Read the model definition and answer for the solid it produces. Units are mm, in the model's axes. Face numbers are marked on the shaded views. A direction names the side the tool comes from. Coordinates: 2 decimals unless noted, no trailing zeros. Order: outer loops, then holes, each group sorted by start corner. A loop starts at its lowest first (then second) coordinate and runs counter-clockwise, first axis right, second up. Notation, with made-up numbers: (28, -3) - (65, -3) arc R21 ccw to (65, 26) - close; hole circle Ø3 at (-29, 48). An arc over 180 degrees is marked (long way). Use one line per item in the form item = value. Start each with the question number.
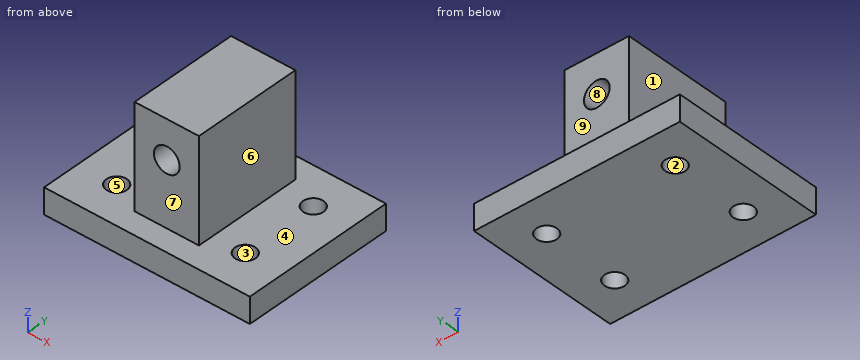
from build123d import *

# Parameters (mm, degrees)
F0_W     = 50.8
F0_H     = 38.1
F1_DEPTH = 6.35
F2_W     = 15.875
F2_H     = 27
F3_DEPTH = 25.4
F4_R     = 3.175
F5_DEPTH = 32.551
F7_D     = 5.0546


with BuildPart() as f1:
    # F0 (on Top) → F1 (new body)
    with BuildSketch(Plane.XY):
        Rectangle(F0_W, F0_H)
    extrude(amount=F1_DEPTH)

    # F2 (on face) → F3 (join)
    with BuildSketch(Plane.XY.offset(6.35)):
        Rectangle(F2_W, F2_H)
    extrude(amount=F3_DEPTH)

    # F4 (on face) → F5 (cut, through all)
    with BuildSketch(Plane.XZ.offset(13.5)):
        with Locations((0, 22.225)):
            Circle(F4_R)
    extrude(amount=-F5_DEPTH, mode=Mode.SUBTRACT)

    # F7 (through all)
    with Locations(Plane.XY.offset(6.35)):
        with Locations((-15.875, 9.525), (-15.875, -9.525), (15.875, 9.525), (15.875, -9.525)):
            Hole(F7_D / 2)


solid = f1.part
Q1. Which of the six approach directions +Z, -Z, +X, -X, +Y, -Y give full straight-line access (tool end or side, diameter ignored) to the marked faces 5, 6, 7, 8 and 9?
Q2. A cutting plane is placed at A-A (x = 0). Give the vertices of the cut face in (y, z).
Q3. A cutting plane is placed at C-C (z = 2). Give the vertices of the cut face in (x, y) (3 decimals), then the cut area to 3 significant figures.
Q4. Given P1, Ø4.5, axis at x = -15.875, y = -9.525, coming from the +Z side; P2, Ø8, axis at x = -2, z = 16, coming from the +Y side; P3, Ø8.5, axis at x = 0, z = 22.225, coming from the -Y side; P4, Ø3, axis at x = 14, y = 1.5, coming from the +Z side, each flat-ended and moving along its own axis, determine where each tip first touches the part or whether it passes through.
Q5. A cutting plane is placed at B-B (y = 8.5). Give the number of separate pieces and of enclosed holes in the cut face, then the cut area to 3 significant figures.
Q6. For a pull along X with two mould halves and no side action, classify the marked faces 1, 2, 3 and 4 as +X half, -X half, draft (parallel to the pull), parting line (faces both ways), or undercut.
Q7. Consider probe 1 along Z at (x, y) = (0, -1); probe 2 along X at (y, z) = (3.5, 12.5); probe 3 along Y at (x, z) = (-5, 8.5). Determine where each line is inside the solid, lowest interval first.
Q8. A cutting plane is placed at D-D (y = -15). Give the vertices of the cut face in (x, z), then the cut area to 3 significant figures.
Result sheet:
q1.face_5 = +Z, -Z
q1.face_6 = +Z, +X, +Y, -Y
q1.face_7 = +Z, +X, -X, -Y
q1.face_8 = +Y, -Y
q1.face_9 = +Z, +X, -X, +Y
q2.outline = (-19.05, 0) - (19.05, 0) - (19.05, 6.35) - (13.5, 6.35) - (13.5, 19.05) - (-13.5, 19.05) - (-13.5, 6.35) - (-19.05, 6.35) - close; (-13.5, 25.4) - (13.5, 25.4) - (13.5, 31.75) - (-13.5, 31.75) - close
q3.outline = (-25.4, -19.05) - (25.4, -19.05) - (25.4, 19.05) - (-25.4, 19.05) - close; hole circle Ø5.055 at (-15.875, -9.525); hole circle Ø5.055 at (-15.875, 9.525); hole circle Ø5.055 at (15.875, -9.525); hole circle Ø5.055 at (15.875, 9.525)
q3.area = 1,860 mm^2
q4.P1 = through
q4.P2 = 13.5
q4.P3 = -13.5
q4.P4 = 6.35
q5.separate_pieces = 3
q5.enclosed_holes = 1
q5.area = 635 mm^2
q6.face_1 = -X half
q6.face_2 = undercut
q6.face_3 = undercut
q6.face_4 = draft
q7.probe_1 = 0 to 19.05, 25.4 to 31.75
q7.probe_2 = -7.94 to 7.94
q7.probe_3 = -13.5 to 13.5
q8.outline = (-25.4, 0) - (25.4, 0) - (25.4, 6.35) - (-25.4, 6.35) - close
q8.area = 323 mm^2
